Geometry: final body of the model. Coordinates: model frame, mm. A direction names the side the tool comes from. Give positions to 0.01 mm unless a question says otherwise; leave off trailing zeros. Write each loop counter-clockwise with the first axis right and the second up, starting at its lowest first coordinate (ties: lowest second). Pieces come first, ordered by that corner, then holes. Notation, with made-up numbers: (58, 12) - (101, 12) arc R31 ccw to (101, 44) - close; hole circle Ø9 at (37.25, 9.25). An arc over 180 degrees is marked (long way). Use CSV: the item, a comma, the result in double quotes. Start each with the question number.
(1) Section C-C on x = 0. Output: boundary loops of the cut face in (y, z).
(2) Section B-B on z = -5.25. Output: boundary loops of the cut face in (x, y), and give its area (3 significant figures).
(3) Reachability of faces 4 (the cylindrical face through (39.463, 0.088, -4.93)), 5 (the flat face through (21.37, 10.19, -4.93)) from +Z, -Z, +X, -X, +Y, -Y: full face, straight path, thin tool, end or side. Return the list, or none.
(4) Line query: probe 1 along Y at (x, z) = (0, -4.75); probe 2 along Y at (x, z) = (3, -3); probe 3 along X at (y, z) = (0.5, -3.5). Output: solid intervals per line, ascending. Write a range as [from, to].
(5) Section A-A on y = 0. Output: boundary loops of the cut face in (x, z), and give its area (3 significant figures).
(6) First-contact query: pin 1 Ø1 at (x, z) = (12, -3.5) entering from +Y; pin 2 Ø3 at (y, z) = (10.5, -1.5) entering from +X; pin 3 Ø6 at (y, z) = (-4.5, -8.5) entering from +X. Flat tips, straight axial feed; report the tip coordinate or a pass-through.
(7) Draft query along X for faces 1 (the flat face through (22.33, -11.27, -4.93)), 2 (the cylindrical face through (38.083, 0.066, -4.93)), 3 (the flat face through (12, 15, -10)). Return one class per face: released by +X, released by -X, zero draft, split by the parting line, or undercut.
from build123d import *

# Parameters (mm, degrees)
EXTRUDE_1_DEPTH = 10


with BuildPart() as part:
    # Эскиз1 → Бобышка-Вытянуть1 (new body)
    with BuildSketch(Plane.XY):
        with BuildLine():
            Line((8.019912069, 17.740535298), (36.250564664, 4.978386487))
            ThreePointArc((36.250564664, 4.978386487), (39.463458, 0), (36.250564664, -4.978386487))
            Line((36.250564664, -4.978386487), (8.019912069, -17.740535298))
            ThreePointArc((8.019912069, -17.740535298), (-19.469093, 0), (8.019912069, 17.740535298))
        make_face()
        with BuildLine():
            Line((35.682100655, -3.720909381), (7.45144806, -16.483058192))
            ThreePointArc((7.45144806, -16.483058192), (-18.089093, 0), (7.45144806, 16.483058192))
            Line((7.45144806, 16.483058192), (35.682100655, 3.720909381))
            ThreePointArc((35.682100655, 3.720909381), (38.083458, 0), (35.682100655, -3.720909381))
        make_face(mode=Mode.SUBTRACT)
    extrude(amount=-EXTRUDE_1_DEPTH)


solid = part.part
Check values:
1,outline,"(-19.47, -10) - (-18.09, -10) - (-18.09, 0) - (-19.47, 0) - close; (18.09, -10) - (19.47, -10) - (19.47, 0) - (18.09, 0) - close"
2,outline,"(8.02, -17.74) - (36.25, -4.98) arc R5.46 ccw to (36.25, 4.98) - (8.02, 17.74) arc R19.47 ccw (long way) to start; hole (7.45, -16.48) - (35.68, -3.72) arc R4.08 ccw to (35.68, 3.72) - (7.45, 16.48) arc R18.09 ccw (long way) to start"
2,area,"204 mm²"
3,face 4,"+Z, -Z, +X"
3,face 5,"+Z, -Z"
4,probe 1,"y = [-19.47, -18.09], [18.09, 19.47]"
4,probe 2,"y = [-19.24, -17.84], [17.84, 19.24]"
4,probe 3,"x = [-19.46, -18.08], [38.05, 39.44]"
5,outline,"(-19.47, -10) - (-18.09, -10) - (-18.09, 0) - (-19.47, 0) - close; (38.08, -10) - (39.46, -10) - (39.46, 0) - (38.08, 0) - close"
5,area,"27.6 mm²"
6,pin 1,"stops at y = 16.17"
6,pin 2,"stops at x = 27.35"
6,pin 3,"stops at x = 39.25"
7,face 1,"released by +X"
7,face 2,"undercut"
7,face 3,"zero draft"
